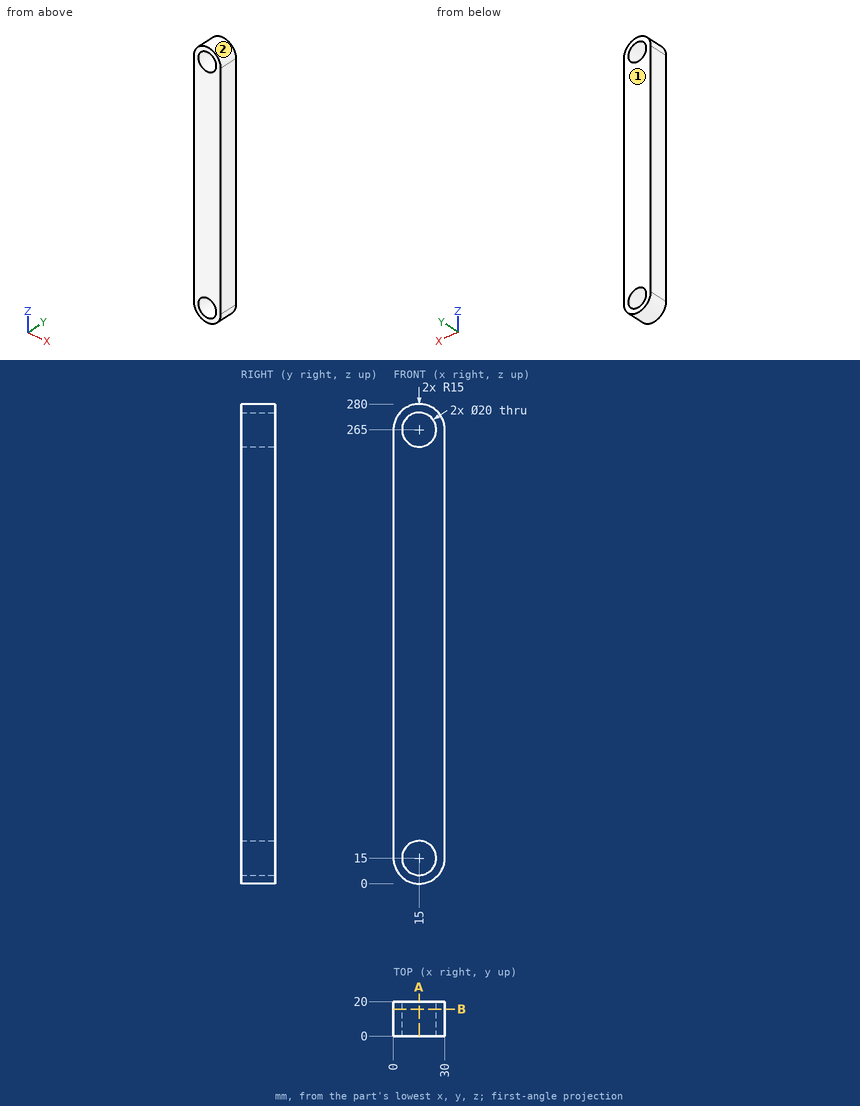
Verification items for this drawing (mm, ordinates from the low corner). Round coordinates to 2 decimals unless told otherwise and drop trailing zeros. Write each loop counter-clockwise with the first axis right and the second up, starting at its lowest first coordinate (ties: lowest second). Pieces come first, ordered by that corner, then holes. Notation, with made-up numbers: M 85.25,79.25 L 109.25,79.25 A18 ccw 109.25,93.25 Z; hole C 58,-29.5 d4. An arc over 180 degrees is marked long. Write item = value, one per line. Start each with the question number.
1. Scan lines: line 1 (Z direction, x = 15, y = 12); line 2 (Z direction, x = 22, y = 10.5); line 3 (Z direction, x = 26, y = 18). Record each from-to range of solid material in increasing order. Write a range as [from, to].
2. Release check for a two-part mould opening along X. For the marked faces 1 and 2 record: pulls with the +X half, pulls with the -X half, needs draft (parallel to the pull), parting line crosses it, or undercut.
3. Section check B-B, the plane y = 15.75. Record the cut outline in (x, z).
4. Gauge pin test, flat ends, axial feed: pin 1 (4 mm diameter, centred on x = 10.5, y = 16, fed in from -Z); pin 2 (12 mm diameter, centred on x = 15, z = 265, fed in from +Y); pin 3 (12 mm diameter, centred on x = 3.5, y = 7.5, fed in from +Z); pin 4 (12 mm diameter, centred on x = 4, y = 15, fed in from +Z). Record the tip position at first contact, or that the pin passes through.
5. Section check A-A, the plane x = 15. Record the cut outline in (y, z).
Results found:
q1.line_1 = [0, 5], [25, 255], [275, 280]
q1.line_2 = [1.73, 7.86], [22.14, 257.86], [272.14, 278.27]
q1.line_3 = [4.8, 275.2]
q2.face_1 = needs draft
q2.face_2 = parting line crosses it
q3.outline = M 0,15 A15 ccw 30,15 L 30,265 A15 ccw 0,265 Z; hole C 15,15 d20; hole C 15,265 d20
q4.pin_1 = 0.21
q4.pin_2 = through
q4.pin_3 = 278.96
q4.pin_4 = 279.14
q5.outline = M 0,0 L 20,0 L 20,5 L 0,5 Z; M 0,25 L 20,25 L 20,255 L 0,255 Z; M 0,275 L 20,275 L 20,280 L 0,280 Z
